Here's the drawing with two shaded views (mm, measured from the low corner). I have some questions. Round coordinates to 2 decimals unless told otherwise and drop trailing zeros. Loops run counter-clockwise (first coordinate to the right, second up) from the corner with the lowest first, then second, coordinate; pieces in that order, holes last. Notation, with made-up numbers: M 88,59.25 L 101,59.25 A16 cw 101,82.25 Z; hole C 21.25,64 d9. An arc over 180 degrees is marked long. One line per item, written item: value. Start each with the question number.
Q1. Imagine slicing it at D-D (y = 40). Please give me the cut outline in (x, z), then the cut area to 3 significant figures.
Q2. I'm going to push flat-ended pins straight in: pin 1 Ø2.5 at (x, y) = (35, 20) entering from +Z; pin 2 Ø6 at (x, y) = (45.5, 26) entering from +Z; pin 3 Ø8 at (x, z) = (35.5, 19.5) entering from +Y; pin 4 Ø10 at (y, z) = (48.5, 56) entering from -X. Where does each tip first touch, or does it pass through?
Q3. Imagine slicing it at A-A (x = 10). Please give me the cut outline in (y, z), then the cut area to 3 significant figures.
Q4. Thinking about a two-plate mould opening in Z: for the marked faces 1, 2 and 3, which applies, released by +Z, released by -Z, zero draft, split by the parting line, or undercut?
Q5. Please list where these lines run through material, in increasing order: line 1 along X through (y, z) = (70, 2.65); line 2 along X through (y, z) = (20, 2.1); line 3 along Y through (x, z) = (45, 2.05).
Q6. Imagine slicing it at C-C (x = 45). Please give me the cut outline in (y, z).
Q7. Imagine slicing it at B-B (y = 10). Please give me the cut outline in (x, z).
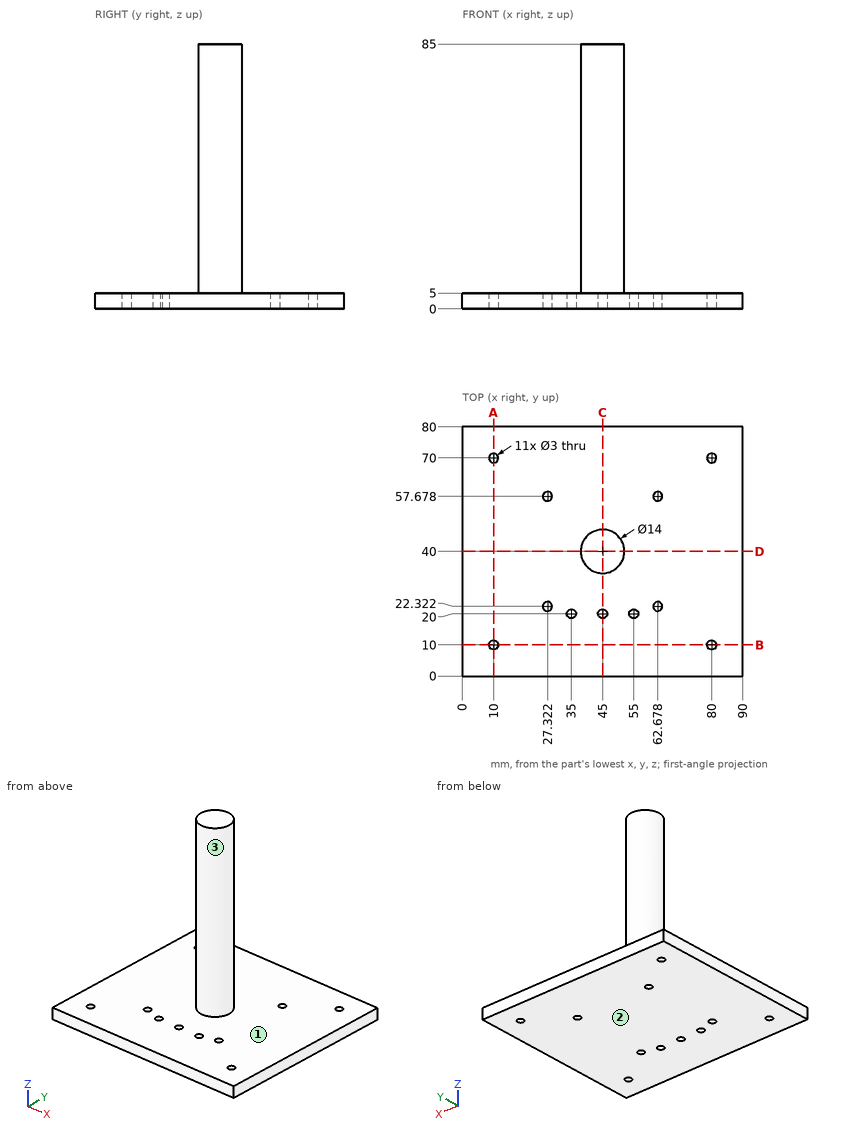
Report:
1. outline: M 0,0 L 90,0 L 90,5 L 52,5 L 52,85 L 38,85 L 38,5 L 0,5 Z
1. area: 1,570 mm²
2. pin 1: passes through
2. pin 2: stops at z = 5
2. pin 3: stops at y = 44.33
2. pin 4: stops at x = 38.94
3. outline: M 0,0 L 8.5,0 L 8.5,5 L 0,5 Z; M 11.5,0 L 68.5,0 L 68.5,5 L 11.5,5 Z; M 71.5,0 L 80,0 L 80,5 L 71.5,5 Z
3. area: 370 mm²
4. face 1: released by +Z
4. face 2: released by -Z
4. face 3: zero draft
5. line 1: x = 0 to 8.5, 11.5 to 78.5, 81.5 to 90
5. line 2: x = 0 to 33.5, 36.5 to 43.5, 46.5 to 53.5, 56.5 to 90
5. line 3: y = 0 to 18.5, 21.5 to 80
6. outline: M 0,0 L 18.5,0 L 18.5,5 L 0,5 Z; M 21.5,0 L 80,0 L 80,5 L 47,5 L 47,85 L 33,85 L 33,5 L 21.5,5 Z
7. outline: M 0,0 L 8.5,0 L 8.5,5 L 0,5 Z; M 11.5,0 L 78.5,0 L 78.5,5 L 11.5,5 Z; M 81.5,0 L 90,0 L 90,5 L 81.5,5 Z
